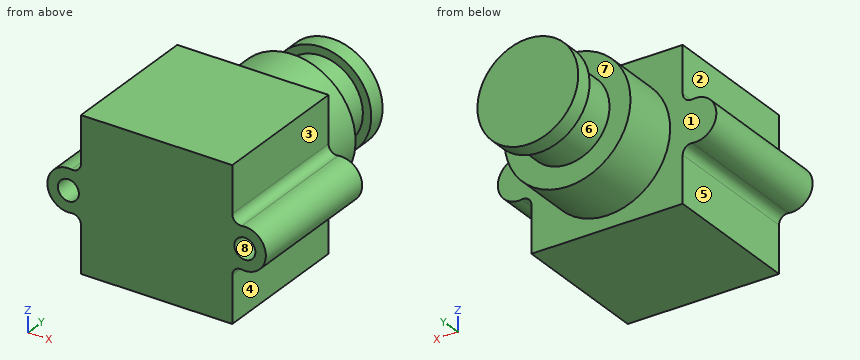
from build123d import *

# Parameters (mm, degrees)
SKETCH1_W           = 18
SKETCH1_H           = 18
BOSS_EXTRUDE1_DEPTH = 17
SKETCH2_R           = 7.5
BOSS_EXTRUDE2_DEPTH = 7
SKETCH3_R           = 5
BOSS_EXTRUDE3_DEPTH = 5
SKETCH4_R           = 6
BOSS_EXTRUDE4_DEPTH = 2
SKETCH5_R           = 2.5
BOSS_EXTRUDE5_DEPTH = 17
FILLET1_R           = 1
SKETCH6_R           = 1.25
CUT_EXTRUDE1_DEPTH  = 6


with BuildPart() as part:
    # Sketch1 → Boss-Extrude1 (new body)
    with BuildSketch(Plane(origin=(0, 0, 0), x_dir=(1, 0, 0), z_dir=(0, 1, 0))):
        Rectangle(SKETCH1_W, SKETCH1_H)
    extrude(amount=BOSS_EXTRUDE1_DEPTH)

    # Sketch2 → Boss-Extrude2 (add)
    with BuildSketch(Plane(origin=(0, 17, 0), x_dir=(1, 0, 0), z_dir=(0, 1, 0))):
        with Locations(Location((0, 0, 0), (0, 0, 90))):
            Circle(SKETCH2_R)
    extrude(amount=BOSS_EXTRUDE2_DEPTH)

    # Sketch3 → Boss-Extrude3 (add)
    with BuildSketch(Plane(origin=(0, 24, 0), x_dir=(1, 0, 0), z_dir=(0, 1, 0))):
        with Locations(Location((0, 0, 0), (0, 0, 270))):
            Circle(SKETCH3_R)
    extrude(amount=BOSS_EXTRUDE3_DEPTH)

    # Sketch4 → Boss-Extrude4 (add)
    with BuildSketch(Plane(origin=(0, 29, 0), x_dir=(1, 0, 0), z_dir=(0, 1, 0))):
        with Locations(Location((0, 0, 0), (0, 0, 270))):
            Circle(SKETCH4_R)
    extrude(amount=BOSS_EXTRUDE4_DEPTH)

    # Sketch5 → Boss-Extrude5 (add)
    with BuildSketch(Plane.XZ):
        with Locations((-10.5, 0)):
            Circle(SKETCH5_R)
        with Locations((10.5, 0)):
            Circle(SKETCH5_R)
    extrude(amount=-BOSS_EXTRUDE5_DEPTH)

    # Fillet1
    fillet1_edges = [part.edges().sort_by_distance(p)[0] for p in [
        (-9, 8.5, 2),
        (-9, 8.5, -2),
        (9, 8.5, -2),
        (9, 8.5, 2),
    ]]
    fillet(fillet1_edges, radius=FILLET1_R)

    # Sketch6 → Cut-Extrude1 (cut)
    with BuildSketch(Plane.XZ):
        with Locations(Location((-10.5, 0, 0), (0, 0, 270))):
            Circle(SKETCH6_R)
        with Locations(Location((10.5, 0, 0), (0, 0, 270))):
            Circle(SKETCH6_R)
    extrude(amount=-CUT_EXTRUDE1_DEPTH, mode=Mode.SUBTRACT)


solid = part.part
Input: part model. Units: mm. Frame: model coordinates. Face numbers are marked on the shaded views. A direction names the side the tool comes from. Round coordinates to 2 decimals unless told otherwise and drop trailing zeros. Order: outer loops, then holes, each group sorted by start corner. A loop starts at its lowest first (then second) coordinate and runs counter-clockwise, first axis right, second up. Notation, with made-up numbers: (55, 54.5) - (77, 54.5) arc R15 cw to (77, 73.5) - close; hole circle Ø11 at (45.5, -23.5). An arc over 180 degrees is marked (long way). Answer as a JSON object with one key per item and string values. Group by question number.
(1) Cut plane D-D (z = 4). Return loops of the section in (x, y).
(2) Draft query along X for the marked faces 6, 7 and 8. Return one class per face: released by +X, released by -X, zero draft, split by the parting line, or undercut.
(3) Pin query (flat end, axial travel): P1, Ø3, axis at x = 10, z = 0, coming from the -Y side; P2, Ø6, axis at y = 7, z = 7.5, coming from the -X side; P3, Ø3, axis at x = -10.5, z = 0, coming from the +Y side; P4, Ø4, axis at y = 23.5, z = -7, coming from the -X side. Return the tip coordinate at first contact, or that it passes through.
(4) Cut plane B-B (z = 0). Return loops of the section in (x, y).
(5) Material intervals for probe 1 along X at (y, z) = (2.5, 0); probe 2 along Y at (x, z) = (5.25, 2.25); probe 3 along Y at (x, z) = (8, -3.5), sorted ascending. Write a range as from..to.
(6) Reachability of the marked faces 1, 2, 3, 4 and 5 from +Z, -Z, +X, -X, +Y, -Y: full face, straight path, thin tool, end or side. Return the list, or none.
(7) Cut plane C-C (y = 24.5). Return loops of the section in (x, z).
(8) Cut plane A-A (x = -10.5). Return loops of the section in (y, z), then the cut area to 3 significant figures.
Here are the results:
{
 "1": {"outline": "(-9, 0) - (9, 0) - (9, 17) - (6.34, 17) - (6.34, 24) - (3, 24) - (3, 29) - (4.47, 29) - (4.47, 31) - (-4.47, 31) - (-4.47, 29) - (-3, 29) - (-3, 24) - (-6.34, 24) - (-6.34, 17) - (-9, 17) - close"},
 "2": {"face 6": "split by the parting line", "face 7": "zero draft", "face 8": "undercut"},
 "3": {"P1": "stops at y = 0", "P2": "stops at x = -9", "P3": "stops at y = 17", "P4": "stops at x = -5.59"},
 "4": {"outline": "(-13, 0) - (-11.75, 0) - (-11.75, 6) - (-9.25, 6) - (-9.25, 0) - (9.25, 0) - (9.25, 6) - (11.75, 6) - (11.75, 0) - (13, 0) - (13, 17) - (7.5, 17) - (7.5, 24) - (5, 24) - (5, 29) - (6, 29) - (6, 31) - (-6, 31) - (-6, 29) - (-5, 29) - (-5, 24) - (-7.5, 24) - (-7.5, 17) - (-13, 17) - close"},
 "5": {"probe 1": "x = -13..-11.75, -9.25..9.25, 11.75..13", "probe 2": "y = 0..24, 29..31", "probe 3": "y = 0..17"},
 "6": {"face 1": "+Y", "face 2": "+Z, -X, +Y, -Y", "face 3": "+Z, +X, +Y, -Y", "face 4": "-Z, +X, +Y, -Y", "face 5": "-Z, -X, +Y, -Y"},
 "7": {"outline": "circle Ø10 at (0, 0)"},
 "8": {"outline": "(0, -2.5) - (17, -2.5) - (17, 2.5) - (0, 2.5) - (0, 1.25) - (6, 1.25) - (6, -1.25) - (0, -1.25) - close", "area": "70.0 mm^2"}
}
